```python
from build123d import *

# Parameters (mm, degrees)
SKETCH1_R           = 4
BOSS_EXTRUDE1_DEPTH = 36
SKETCH2_R           = 2.6
CUT_EXTRUDE1_DEPTH  = 4.2
CUT_EXTRUDE2_START  = -10
CUT_EXTRUDE2_DEPTH  = 11.1
CUT_EXTRUDE3_DEPTH  = 5
BOSS_EXTRUDE2_DEPTH = 11.1


with BuildPart() as part:
    # Sketch1 → Boss-Extrude1 (new body)
    with BuildSketch(Plane.XY):
        with BuildLine():
            Line((-14.75, -7.9), (-14.75, -12))
            Line((-14.75, -12), (-23.75, -12))
            Line((-23.75, -12), (-23.75, -7.9))
            ThreePointArc((-23.75, -7.9), (-21.521408325, -4.313621249), (-17.318943727, -4.723529412))
            ThreePointArc((-17.318943727, -4.723529412), (-12.846321275, -2.097250623), (-17.881535856, -0.852941176))
            ThreePointArc((-17.881535856, -0.852941176), (-24.891297515, 0.177367286), (-20.057391817, 5.357294867))
            ThreePointArc((-20.057391817, 5.357294867), (-17.669207765, 5.792991841), (-16.519021958, 7.930824279))
            ThreePointArc((-16.519021958, 7.930824279), (-12.452765055, 11.749381379), (-8.523313091, 7.790185654))
            ThreePointArc((-8.523313091, 7.790185654), (-7.626821013, 6.431985616), (-6.020047535, 6.690218806))
            ThreePointArc((-6.020047535, 6.690218806), (0, 9), (6.020047535, 6.690218806))
            ThreePointArc((6.020047535, 6.690218806), (7.626821013, 6.431985616), (8.523313091, 7.790185654))
            ThreePointArc((8.523313091, 7.790185654), (12.452765055, 11.749381379), (16.519021958, 7.930824279))
            ThreePointArc((16.519021958, 7.930824279), (17.669207765, 5.792991841), (20.057391817, 5.357294867))
            ThreePointArc((20.057391817, 5.357294867), (24.891297515, 0.177367286), (17.881535856, -0.852941176))
            ThreePointArc((17.881535856, -0.852941176), (12.846321275, -2.097250623), (17.318943727, -4.723529412))
            ThreePointArc((17.318943727, -4.723529412), (21.521408325, -4.313621249), (23.75, -7.9))
            Line((23.75, -7.9), (23.75, -12))
            Line((23.75, -12), (14.75, -12))
            Line((14.75, -12), (14.75, -7.9))
            Line((14.75, -7.9), (21.994994432, -7.9))
            ThreePointArc((21.994994432, -7.9), (22.385089181, -7.712771621), (22.4830367, -7.291304348))
            ThreePointArc((22.4830367, -7.291304348), (20.708026906, -5.268995544), (18.048260609, -5.676470588))
            ThreePointArc((18.048260609, -5.676470588), (11.658799963, -1.924643747), (18.85196365, -0.147058824))
            ThreePointArc((18.85196365, -0.147058824), (23.758796811, 0.5741571), (20.375062823, 4.200106407))
            ThreePointArc((20.375062823, 4.200106407), (16.963371319, 4.822530655), (15.320248738, 7.876576995))
            ThreePointArc((15.320248738, 7.876576995), (12.581969864, 10.5493813), (9.733766071, 7.99403608))
            Line((9.733766071, 7.99403608), (8.965752283, -0.784401685))
            ThreePointArc((8.965752283, -0.784401685), (0, -9), (-8.965752283, -0.784401685))
            Line((-8.965752283, -0.784401685), (-9.733766071, 7.99403608))
            ThreePointArc((-9.733766071, 7.99403608), (-12.581969864, 10.5493813), (-15.320248738, 7.876576995))
            ThreePointArc((-15.320248738, 7.876576995), (-16.963371319, 4.822530655), (-20.375062823, 4.200106407))
            ThreePointArc((-20.375062823, 4.200106407), (-23.758796811, 0.5741571), (-18.85196365, -0.147058824))
            ThreePointArc((-18.85196365, -0.147058824), (-11.658799963, -1.924643747), (-18.048260609, -5.676470588))
            ThreePointArc((-18.048260609, -5.676470588), (-20.708026906, -5.268995544), (-22.4830367, -7.291304348))
            ThreePointArc((-22.4830367, -7.291304348), (-22.385089181, -7.712771621), (-21.994994432, -7.9))
            Line((-21.994994432, -7.9), (-14.75, -7.9))
        make_face()
        Circle(SKETCH1_R, mode=Mode.SUBTRACT)
    extrude(amount=BOSS_EXTRUDE1_DEPTH)

    # Sketch2 → Cut-Extrude1 (cut)
    with BuildSketch(Plane.XZ.offset(12)):
        with Locations(Location((-19.225, 30.5, 0), (0, 0, 270))):  # turned: the seam where the file's is
            Circle(SKETCH2_R)
        with Locations(Location((-19.225, 5.5, 0), (0, 0, 270))):  # turned: the seam where the file's is
            Circle(SKETCH2_R)
        with Locations(Location((19.225, 5.5, 0), (0, 0, 270))):  # turned: the seam where the file's is
            Circle(SKETCH2_R)
        with Locations(Location((19.225, 30.5, 0), (0, 0, 270))):  # turned: the seam where the file's is
            Circle(SKETCH2_R)
    extrude(amount=-CUT_EXTRUDE1_DEPTH, mode=Mode.SUBTRACT)

    # Sketch3 → Cut-Extrude2 (cut)
    with BuildSketch(Plane.XY.offset(36).offset(CUT_EXTRUDE2_START)):
        with BuildLine():
            Line((-7.008961202, 7.254714015), (-6.325836333, -0.553438966))
            ThreePointArc((-6.325836333, -0.553438966), (0, -6.35), (6.325836333, -0.553438966))
            Line((6.325836333, -0.553438966), (7.008961202, 7.254714015))
            ThreePointArc((7.008961202, 7.254714015), (0, 10.087438355), (-7.008961202, 7.254714015))
        make_face()
    extrude(amount=-CUT_EXTRUDE2_DEPTH, mode=Mode.SUBTRACT)

    # Sketch4 → Cut-Revolve1 (revolve, cut)
    with BuildSketch(Plane(origin=(0, 0, 0), x_dir=(1, 0, 0), z_dir=(0, 1, 0))):
        Polygon((0, -14.9), (-6.35, -14.9), (-6.35, -30), (-1.273774508, -36.049609967), (0, -36.049609967), align=None)
    revolve(axis=Axis((0, 0, 14.9), (0, 0, 1)), mode=Mode.SUBTRACT)

    # Sketch5 → Cut-Extrude3 (cut)
    with BuildSketch(Plane.XY.offset(14.9)):
        Polygon((5.35, -3.08882394), (5.35, 3.08882394), (0, 6.17764788), (-5.35, 3.08882394), (-5.35, -3.08882394), (0, -6.17764788), align=None)
    extrude(amount=-CUT_EXTRUDE3_DEPTH, mode=Mode.SUBTRACT)

    # Sketch6 → Boss-Extrude2 (add)
    with BuildSketch(Plane.XY.offset(14.9)):
        with BuildLine():
            Line((-4.466040087, 6.877098657), (-4.19372057, 6.457763373))
            ThreePointArc((-4.19372057, 6.457763373), (0, 7.7), (4.19372057, 6.457763373))
            Line((4.19372057, 6.457763373), (4.466040087, 6.877098657))
            ThreePointArc((4.466040087, 6.877098657), (0, 8.2), (-4.466040087, 6.877098657))
        make_face()
    extrude(amount=BOSS_EXTRUDE2_DEPTH)


solid = part.part
```
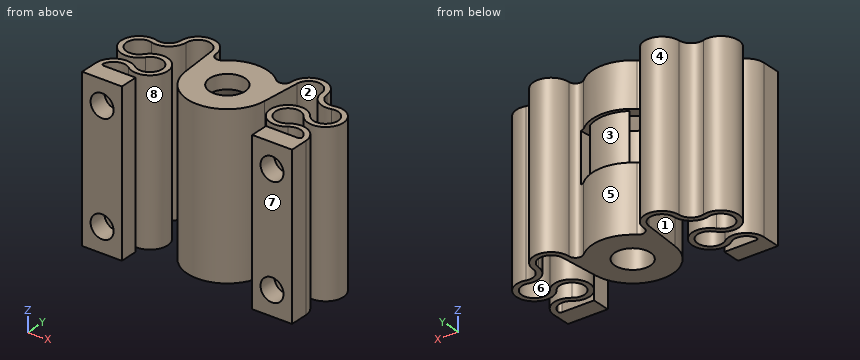
Design review of the part built by this model. Coordinates are the model's own, in mm. Face numbers are marked on the shaded views. A direction names the side the tool comes from. Coordinates: 2 decimals unless noted, no trailing zeros. Order: outer loops, then holes, each group sorted by start corner. A loop starts at its lowest first (then second) coordinate and runs counter-clockwise, first axis right, second up.
1) For the marked faces 1, 2, 3 and 4, list the 3-axis set-ups (+Z, -Z, +X, -X, +Y, -Y) from which the entire face can be reached by the end or side of a thin tool; tool diameter is ignored.
2) Take a section at A-A, the plane z = 31. State how many separate pieces and enclosed holes the cut face has, and give its area (3 significant figures).
3) Mouldability with a two-part tool opening along Y and no side actions: class the marked faces 5, 6, 7 and 8 as +Y half, -Y half, draft (parallel to the pull), parting line (faces both ways), or undercut.
4) Take a section at C-C, the plane x = 7.5. Give the boundary of the cut face in (y, z).
5) Wall thickness on line 1 along X through (y, z) = (-9.15, 30.5) (3 decimals); line 2 along Y through (x, z) = (-14, 4.5); line 3 along Y through (x, z) = (0, 7.5): over which ranges is each line inside the solid? List them lowest first.
6) Clearance check with flat-ended pins moving along their axes: pin 1 (3.5 mm diameter, centred on y = -10.5, z = 14, fed in from +X); pin 2 (5 mm diameter, centred on x = -20, z = 6, fed in from +Y); pin 3 (4.5 mm diameter, centred on x = -19.225, z = 5.5, fed in from -Y). State where each tip first meets the part, or that it passes through.
Returned:
1. face 1: +Z, -Z, -Y
1. face 2: +Z, -Z
1. face 3: +Y
1. face 4: +Z, -Z, +Y
2. separate pieces: 3
2. enclosed holes: 1
2. area: 342 mm2
3. face 5: +Y half
3. face 6: undercut
3. face 7: -Y half
3. face 8: undercut
4. outline: (-4.97, 0) - (6.38, 0) - (6.38, 36) - (-4.97, 36) - close
5. line 1: x = -23.75 to -21.825, -16.625 to -14.75, 14.75 to 16.625, 21.825 to 23.75
5. line 2: y = -6.16 to -4.79, -0.21 to 1.16, 10.13 to 11.47
5. line 3: y = -9 to -4, 4 to 9
6. pin 1: stops at x = 23.75
6. pin 2: stops at y = 5.93
6. pin 3: stops at y = -6.26
